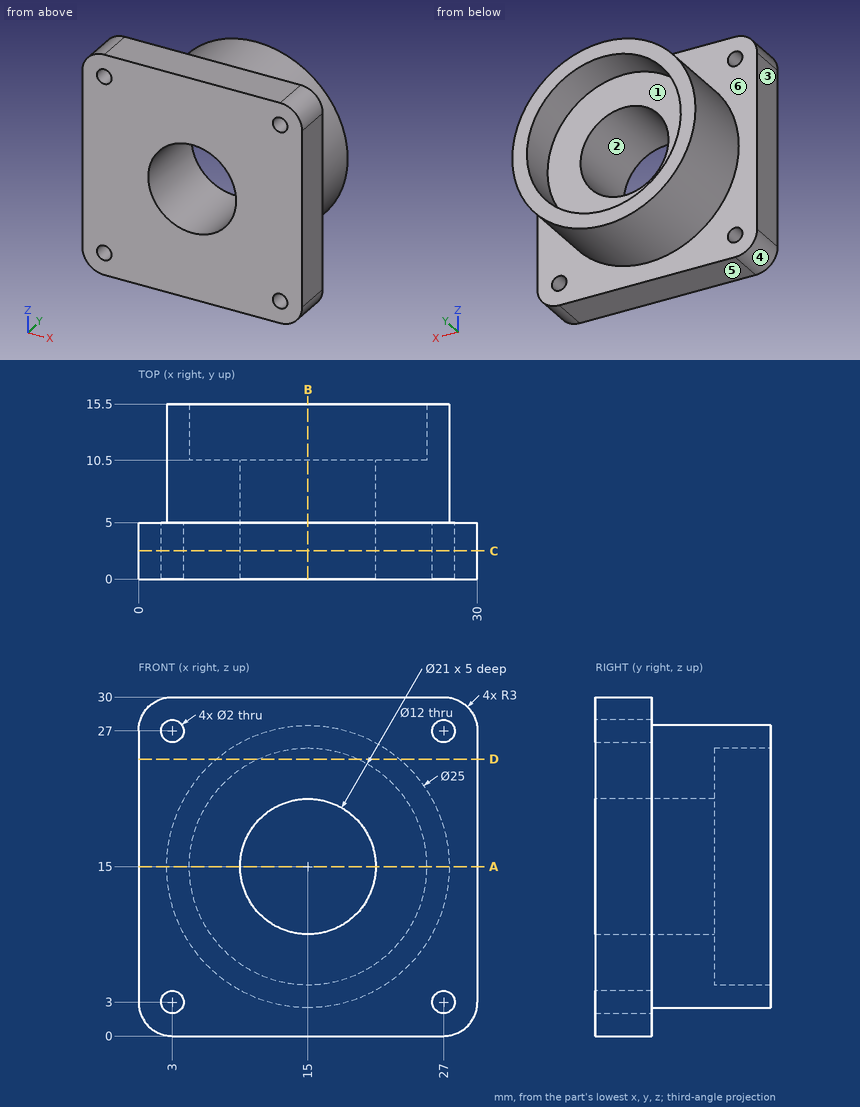
Verification items for this drawing (mm, ordinates from the low corner). A direction names the side the tool comes from. Give positions to 0.01 mm unless a question says otherwise; leave off trailing zeros. Loops run counter-clockwise (first coordinate to the right, second up) from the corner with the lowest first, then second, coordinate; pieces in that order, holes last. Notation, with made-up numbers: M 9,12.5 L 48,12.5 A21 cw 48,39.5 Z; hole C 54,51 d4. An arc over 180 degrees is marked long. Return JSON: item names as keys, results as strings. Group by question number.
1. Mould release check, pull along Z, two halves, no side actions. Record for the marked faces 1, 2, 3 and 4: released by +Z, released by -Z, zero draft, split by the parting line, or undercut.
2. Cross-section at A-A on z = 15. Record the boundary of the cut face in (x, y), plus the area to 4 significant figures.
3. Tool access check on the marked faces 5 and 6. Record the directions out of +Z, -Z, +X, -X, +Y, -Y that give a thin tool (end or side, any length) a straight path to the whole face; none if there is none.
4. Cross-section at D-D on z = 24.5. Record the boundary of the cut face in (x, y), plus the area to 3 significant figures.
5. Cross-section at C-C on y = 2.5. Record the boundary of the cut face in (x, z).
6. Thickness scan on L1, parallel to X at y = 1.4, z = 27; L2, parallel to X at y = 5.25, z = 15; L3, parallel to X at y = 11.25, z = 15.25. Record the ranges inside material, lowest first.
7. Cross-section at B-B on x = 15. Record the boundary of the cut face in (y, z).
8. Go/stop test with flat-tipped pins: pin 1 (3 mm diameter, centred on y = 13.5, z = 19, fed in from -X); pin 2 (17 mm diameter, centred on x = 10.5, z = 15, fed in from +Y); pin 3 (2.5 mm diameter, centred on x = 3, z = 3, fed in from +Y); pin 4 (4 mm diameter, centred on x = 17.5, y = 10, fed in from -Z). Record where each tip stops, or that it passes through.
Return value:
{
 "1": {"face 1": "undercut", "face 2": "undercut", "face 3": "zero draft", "face 4": "released by -Z"},
 "2": {"outline": "M 0,0 L 9,0 L 9,10.5 L 4.5,10.5 L 4.5,15.5 L 2.5,15.5 L 2.5,5 L 0,5 Z; M 21,0 L 30,0 L 30,5 L 27.5,5 L 27.5,15.5 L 25.5,15.5 L 25.5,10.5 L 21,10.5 Z", "area": "181.5 mm^2"},
 "3": {"face 5": "-Z, +X, -X, +Y, -Y", "face 6": "+Y"},
 "4": {"outline": "M 0,0 L 30,0 L 30,5 L 23.12,5 L 23.12,15.5 L 19.47,15.5 L 19.47,10.5 L 10.53,10.5 L 10.53,15.5 L 6.88,15.5 L 6.88,5 L 0,5 Z", "area": "276 mm^2"},
 "5": {"outline": "M 0,3 A3 ccw 3,0 L 27,0 A3 ccw 30,3 L 30,27 A3 ccw 27,30 L 3,30 A3 ccw 0,27 Z; hole C 3,3 d2; hole C 3,27 d2; hole C 15,15 d12; hole C 27,3 d2; hole C 27,27 d2"},
 "6": {"L1": "0 to 2, 4 to 26, 28 to 30", "L2": "2.5 to 9, 21 to 27.5", "L3": "2.5 to 4.5, 25.5 to 27.5"},
 "7": {"outline": "M 0,0 L 5,0 L 5,2.5 L 15.5,2.5 L 15.5,4.5 L 10.5,4.5 L 10.5,9 L 0,9 Z; M 0,21 L 10.5,21 L 10.5,25.5 L 15.5,25.5 L 15.5,27.5 L 5,27.5 L 5,30 L 0,30 Z"},
 "8": {"pin 1": "x = 2.75", "pin 2": "y = 15.5", "pin 3": "y = 5", "pin 4": "z = 2.51"}
}
